Work out the finished part from the listing and answer in its coordinate system (mm). A direction names the side the tool comes from. Give positions to 0.01 mm unless a question says otherwise; leave off trailing zeros. Loops run counter-clockwise (first coordinate to the right, second up) from the corner with the lowest first, then second, coordinate; pieces in that order, holes last. Notation, with made-up numbers: (3, 17) - (8, 17) arc R17 cw to (8, 23) - close; hole circle Ø11 at (34, 54.5). An arc over 180 degrees is marked (long way). Use CSV: the item, a comma, the result in double quotes.
Autodesk Inventor part; units mm, degrees
ref_plane "YZ Plane" through (0, 0, 0) normal (1, 0, 0) x (0, 1, 0)
ref_plane "XZ Plane" through (0, 0, 0) normal (0, 1, 0) x (-1, 0, 0)
ref_plane "XY Plane" through (0, 0, 0) normal (0, 0, 1) x (1, 0, 0)
sketch "Boceto1" plane through (0, 0, 0) normal (0, 1, 0) x (-1, 0, 0)
  circle A0 centre (0, 0) radius 9.9
  dimension "d0" = 19.8
extrude "Extrusión1" add sketch "Boceto1" along normal blind 3.5
sketch "Boceto2" plane through (0, 3.5, 0) normal (0, 1, 0) x (1, 0, 0)
  circle A0 centre (0, 0) radius 9.45
  dimension "d3" = 18.9
extrude "Extrusión2" add sketch "Boceto2" along normal blind 10
sketch "Boceto3" plane through (0, 13.5, 0) normal (0, 1, 0) x (1, 0, 0)
  circle A0 centre (0, 0) radius 5
  dimension "d6" = 10
extrude "Extrusión3" cut sketch "Boceto3" against normal through all
sketch "Boceto4" plane through (0, 13.5, 0) normal (0, 1, 0) x (1, 0, 0)
  circle A0 centre (0, 0) radius 9.45
  circle A1 centre (0, -7.2249) radius 1
  circle A2 centre (0, 7.2249) radius 1
  circle A3 centre (0, 0) radius 5
  circle A4 centre (7.225, 0) radius 1
  circle A5 centre (-7.225, 0) radius 1
  dimension "d9" = 2
  dimension "d10" = 2
extrude "Extrusión4" cut sketch "Boceto4" against normal blind 10 contours A1 | A2 | A4 | A5
properties part number "EejeV2"
Item 1: Given P1, Ø2, axis at x = -2, y = 10.5, coming from the -Z side; P2, Ø1, axis at x = 0, z = -7, coming from the +Y side; P3, Ø5, axis at y = 1.5, z = 3.5, coming from the -X side, each flat-ended and moving along its own axis, determine where each tip first touches the part or whether it passes through.
Determined:
P1,"stops at z = -9.4"
P2,"stops at y = 3.5"
P3,"stops at x = -9.85"
Item 2: A cutting plane is placed at C-C on x = -7.5. Determine the outline of the cut face in (y, z), and give its area (3 significant figures).
Determined:
outline,"(0, -6.46) - (3.5, -6.46) - (3.5, -5.75) - (13.5, -5.75) - (13.5, -0.96) - (3.5, -0.96) - (3.5, 0.96) - (13.5, 0.96) - (13.5, 5.75) - (3.5, 5.75) - (3.5, 6.46) - (0, 6.46) - close"
area,"141 mm²"
Item 3: A cutting plane is placed at D-D on y = 2. Determine the outline of the cut face in (x, z), and give its area (3 significant figures).
Determined:
outline,"circle Ø19.8 at (0, 0); hole circle Ø10 at (0, 0)"
area,"229 mm²"
Item 4: A cutting plane is placed at B-B on x = -0.25. Determine the outline of the cut face in (y, z), and give its area (3 significant figures).
Determined:
outline,"(0, -9.9) - (3.5, -9.9) - (3.5, -9.45) - (13.5, -9.45) - (13.5, -8.19) - (3.5, -8.19) - (3.5, -6.26) - (13.5, -6.26) - (13.5, -4.99) - (0, -4.99) - close; (0, 4.99) - (13.5, 4.99) - (13.5, 6.26) - (3.5, 6.26) - (3.5, 8.19) - (13.5, 8.19) - (13.5, 9.45) - (3.5, 9.45) - (3.5, 9.9) - (0, 9.9) - close"
area,"84.7 mm²"
Item 5: For faces 1 (the cylindrical face through (-0.22, 8.57, 8.2)), 2 (the flat face through (4, 13.5, 4)), determine the directions among +Z, -Z, +X, -X, +Y, -Y from which every point of the face is accessible in a straight line to the end or side of a thin tool.
Determined:
face 1,"+Y"
face 2,"+Z, -Z, +X, -X, +Y"
Item 6: Find the intervals of material crossed by line 1 (Z direction, x = 0, y = 9.5); line 2 (X direction, y = 9, z = 0) (3 decimals); line 3 (X direction, y = 9.75, z = 4), in increasing order.
Determined:
line 1,"z = -9.45 to -8.22, -6.22 to -5, 5 to 6.22, 8.22 to 9.45"
line 2,"x = -9.45 to -8.225, -6.225 to -5, 5 to 6.225, 8.225 to 9.45"
line 3,"x = -8.56 to -3, 3 to 8.56"
Item 7: A cutting plane is placed at A-A on z = 0. Determine the outline of the cut face in (x, y) (3 decimals).
Determined:
outline,"(-9.9, 0) - (-5, 0) - (-5, 13.5) - (-6.225, 13.5) - (-6.225, 3.5) - (-8.225, 3.5) - (-8.225, 13.5) - (-9.45, 13.5) - (-9.45, 3.5) - (-9.9, 3.5) - close; (5, 0) - (9.9, 0) - (9.9, 3.5) - (9.45, 3.5) - (9.45, 13.5) - (8.225, 13.5) - (8.225, 3.5) - (6.225, 3.5) - (6.225, 13.5) - (5, 13.5) - close"
